from build123d import *

# Parameters (mm, degrees)
SKETCH1_R               = 5
BOSS_EXTRUDE1_DEPTH     = 20
BOSS_EXTRUDE2_DEPTH     = 70
CUT_EXTRUDE1_DEPTH      = 146.933344284
CUT_EXTRUDE1_DEPTH_BACK = 146.933344284
SKETCH2_R               = 8
CUT_EXTRUDE2_DEPTH      = 150.013871252
CHAMFER1_SIZE           = 25
CUT_EXTRUDE3_REACH      = 174.264
SKETCH4_W               = 25
SKETCH4_H               = 12


with BuildPart() as part:
    # Sketch1 → Boss-Extrude1 (new body)
    with BuildSketch(Plane(origin=(0, 0, 0), x_dir=(1, 0, 0), z_dir=(0, 1, 0))):
        with BuildLine():
            ThreePointArc((-70.391757976, -55.391757976), (-65.998359694, -65.998359694), (-55.391757976, -70.391757976))
            Line((-55.391757976, -70.391757976), (55.391757976, -70.391757976))
            ThreePointArc((55.391757976, -70.391757976), (65.998359694, -65.998359694), (70.391757976, -55.391757976))
            Line((70.391757976, -55.391757976), (70.391757976, 55.391757976))
            ThreePointArc((70.391757976, 55.391757976), (65.998359694, 65.998359694), (55.391757976, 70.391757976))
            Line((55.391757976, 70.391757976), (-55.391757976, 70.391757976))
            ThreePointArc((-55.391757976, 70.391757976), (-65.998359694, 65.998359694), (-70.391757976, 55.391757976))
            Line((-70.391757976, 55.391757976), (-70.391757976, -55.391757976))
        make_face()
        with Locations(Location((-55.391757976, -55.391757976, 0), (0, 0, 270))):
            Circle(SKETCH1_R, mode=Mode.SUBTRACT)
        with Locations(Location((55.391757976, -55.391757976, 0), (0, 0, 270))):
            Circle(SKETCH1_R, mode=Mode.SUBTRACT)
        with Locations(Location((-55.391757976, 55.391757976, 0), (0, 0, 270))):
            Circle(SKETCH1_R, mode=Mode.SUBTRACT)
        Polygon((42.779960262, -2.474873734), (2.474873734, -42.779960262), (-42.779960262, 2.474873734), (-2.474873734, 42.779960262), align=None, mode=Mode.SUBTRACT)
        with Locations(Location((55.391757976, 55.391757976, 0), (0, 0, 270))):
            Circle(SKETCH1_R, mode=Mode.SUBTRACT)
    extrude(amount=BOSS_EXTRUDE1_DEPTH)

    # Sketch1_3 → Boss-Extrude2 (add)
    with BuildSketch(Plane(origin=(0, 0, 0), x_dir=(1, 0, 0), z_dir=(0, 1, 0))):
        Polygon((-42.779960262, 2.474873734), (-2.474873734, 42.779960262), (42.779960262, -2.474873734), (2.474873734, -42.779960262), align=None)
    extrude(amount=BOSS_EXTRUDE2_DEPTH)

    # Sketch2 → Cut-Extrude1 (cut, two sides: drawn at the far end of the back side and taken through both)
    with BuildSketch(Plane(origin=(20.152543264, 0, -20.152543264), x_dir=(-0.7071067811865475, 0, -0.7071067811865477), z_dir=(0.7071067811865477, 0, -0.7071067811865475)).offset(-CUT_EXTRUDE1_DEPTH_BACK)):
        with Locations(Location((0, 52, 0), (0, 0, 180))):
            Circle(SKETCH2_R)
    extrude(amount=CUT_EXTRUDE1_DEPTH + CUT_EXTRUDE1_DEPTH_BACK, mode=Mode.SUBTRACT)

    # Sketch3 → Cut-Extrude2 (cut, through all)
    with BuildSketch(Plane(origin=(22.627416998, 0, 22.627416998), x_dir=(0.7071067811865475, 0, -0.7071067811865477), z_dir=(0.7071067811865477, 0, 0.7071067811865475))):
        Polygon((16, 40), (16, 70), (-16, 70), (-16, 40), (0, 26), align=None)
    extrude(amount=-CUT_EXTRUDE2_DEPTH, mode=Mode.SUBTRACT)

    # Chamfer1
    chamfer1_edges = [part.edges().sort_by_distance(p)[0] for p in [
        (6.894291117, 70, 38.360542879),
        (38.360542879, 70, 6.894291117),
    ]]
    chamfer(chamfer1_edges, length=CHAMFER1_SIZE)

    # Sketch4 → Cut-Extrude3 (cut, up to next)
    with BuildSketch(Plane(origin=(70.391757976, 0, 0), x_dir=(0, 0, -1), z_dir=(1, 0, 0)), mode=Mode.PRIVATE) as cut_extrude3_sk1:
        Rectangle(SKETCH4_W, SKETCH4_H)
    cut_extrude3_tool1 = extrude(cut_extrude3_sk1.sketch, amount=-CUT_EXTRUDE3_REACH, mode=Mode.PRIVATE) & part.part
    add(cut_extrude3_tool1.solids().sort_by_distance((70.391758, 0, 0))[0], mode=Mode.SUBTRACT)


solid = part.part
Source: CAD feature listing. Evaluate the final solid. Frame: model axes, mm. A direction names the side the tool comes from. Round coordinates to 2 decimals unless told otherwise and drop trailing zeros. Loops run counter-clockwise (first coordinate to the right, second up) from the corner with the lowest first, then second, coordinate; pieces in that order, holes last. Notation, with made-up numbers: (89.5, -3.5) -> (118.5, -3.5) arc R17 ccw to (118.5, 10.5) -> close; hole circle Ø8 at (27.5, -33). An arc over 180 degrees is marked (long way). Answer as a JSON object with one key per item and string values. Group by question number.
Q1. Access query for faces 1 (the flat face through (1, 3, -12.5)), 2 (the flat face through (-18.431, 27.983, -26.824)), 3 (the flat face through (6.6, 58.12, -16.03)). Directions: +Z, -Z, +X, -X, +Y, -Y. A direction counts if a zero-diameter tool reaches every point of the face in a straight line with its end or side. Return the directions, or none.
Q2. Contact query for flat-ended pins moving along their axis: P1, Ø13, axis at x = -55.39, z = 55.39, coming from the -Y side; P2, Ø6, axis at y = 24, z = -25.5, coming from the -X side; P3, Ø1, axis at x = 0.5, y = 40, coming from the -Z side; P4, Ø4, axis at x = -22.5, z = 28, coming from the +Y side. Output: stop coordinate, or through.
Q3. Section query C-C (x = 46). Output: boundary loops of the cut face in (y, z), plus the area to 3 significant figures.
Q4. Mould query, pull axis Z, two halves, no side actions, for faces 4 (the flat face through (19.836, 39.094, -20.469)), 5 (the cylindrical face through (14.93, 44.07, -16.41)), 6 (the flat face through (-1.759, 57.325, 29.584)), 7 (the flat face through (-32, 20, -17)). Classes: pulls with the +Z half, pulls with the -Z half, needs draft (parallel to the pull), parting line crosses it, or undercut.
Q5. Ray query, line 1 (Z direction, x = 20, y = 5); line 2 (X direction, y = 9, z = -51); line 3 (Z direction, x = -12, y = 26.5). Return the intervals inside material, ascending. Write a range as from..to.
Q6. Section query D-D (y = 57). Output: boundary loops of the cut face in (x, z).
Q7. Section query B-B (y = 9.5). Output: boundary loops of the cut face in (x, z), plus the area to 3 significant figures.
Q8. Section query A-A (y = 34.5). Output: boundary loops of the cut face in (x, z).
Completed:
{
 "1": {"face 1": "+X, -X, -Y", "face 2": "-Z, -X, +Y", "face 3": "+Y"},
 "2": {"P1": "y = 0", "P2": "x = -22.75", "P3": "z = -40.31", "P4": "y = 20"},
 "3": {"outline": "(0, -70.39) -> (20, -70.39) -> (20, 70.39) -> (0, 70.39) -> (0, 12.5) -> (6, 12.5) -> (6, -12.5) -> (0, -12.5) -> close", "area": "2,670 mm²"},
 "4": {"face 4": "pulls with the -Z half", "face 5": "undercut", "face 6": "pulls with the +Z half", "face 7": "needs draft"},
 "5": {"line 1": "-70.39..-12.5, 12.5..70.39", "line 2": "-70.39..-57.78, -53..53, 57.78..70.39", "line 3": "-33.25..-12.81, -11.19..28.31"},
 "6": {"outline": "(-42.78, -2.47) -> (-33.94, -11.31) -> (-15.73, 6.9) -> (-24.57, 15.74) -> close; (-15.74, 24.57) -> (-6.9, 15.73) -> (2.83, 25.46) -> (-6.01, 34.29) -> close; (-11.31, -33.94) -> (-2.47, -42.78) -> (15.74, -24.57) -> (6.9, -15.73) -> close; (15.73, -6.9) -> (24.57, -15.74) -> (34.29, -6.01) -> (25.46, 2.83) -> close"},
 "7": {"outline": "(-70.39, -55.39) arc R15 ccw to (-55.39, -70.39) -> (55.39, -70.39) arc R15 ccw to (70.39, -55.39) -> (70.39, 55.39) arc R15 ccw to (55.39, 70.39) -> (-55.39, 70.39) arc R15 ccw to (-70.39, 55.39) -> close; hole circle Ø10 at (-55.39, -55.39); hole circle Ø10 at (-55.39, 55.39); hole circle Ø10 at (55.39, -55.39); hole circle Ø10 at (55.39, 55.39)", "area": "19,300 mm²"},
 "8": {"outline": "(-42.78, -2.47) -> (-29.5, -15.76) -> (15.76, 29.5) -> (2.47, 42.78) -> close; (-15.76, -29.5) -> (-2.47, -42.78) -> (42.78, 2.47) -> (29.5, 15.76) -> close"}
}
